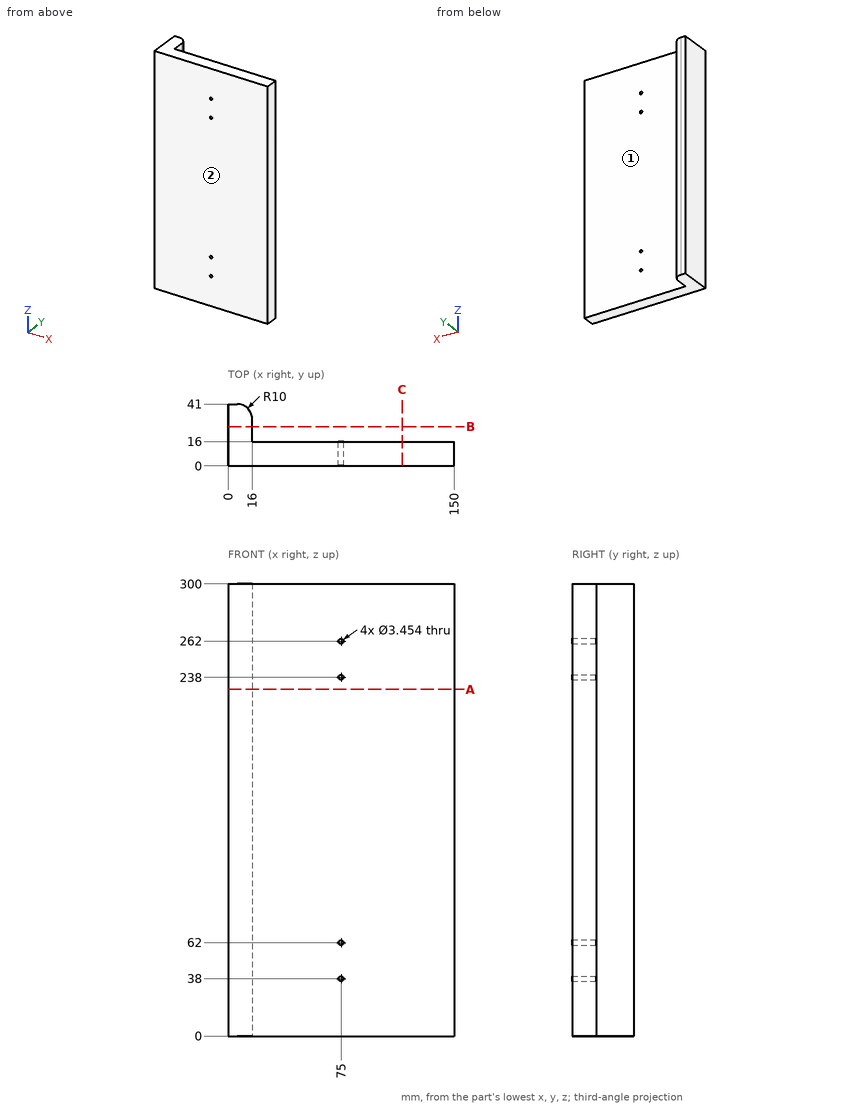
Study the drawing (mm; zero at the part's minimum x, y, z) and answer. A direction names the side the tool comes from. Round coordinates to 2 decimals unless told otherwise and drop trailing zeros. Write each loop counter-clockwise with the first axis right and the second up, starting at its lowest first coordinate (ties: lowest second). Pieces come first, ordered by that corner, then holes. Notation, with made-up numbers: (0.25, 89) -> (4.25, 89) arc R18 ccw to (4.25, 93) -> close; hole circle Ø6 at (13.25, 7.5). An arc over 180 degrees is marked (long way). Write item = value, one per line.
1) Section B-B on y = 26 is taken. Write down the section's boundary in (x, z).
Check values:
outline = (0, 0) -> (16, 0) -> (16, 300) -> (0, 300) -> close
2) Straight lines are drawn through the part: line 1 along Z through (x, y) = (75, 11); line 2 along X through (y, z) = (3, 238); line 3 along Y through (x, z) = (77, 148.5). For each, find the intervals that lie inside material, in ascending order. Write a range as [from, to].
Check values:
line_1 = [0, 36.27], [39.73, 60.27], [63.73, 236.27], [239.73, 260.27], [263.73, 300]
line_2 = [0, 73.27], [76.73, 150]
line_3 = [0, 16]
3) Given pin 1 (5.5 mm diameter, centred on x = 75, z = 62, fed in from +Y); pin 2 (3 mm diameter, centred on y = 29.5, z = 84.5, fed in from +X); pin 3 (2 mm diameter, centred on y = 34.5, z = 174.5, fed in from -X), each flat-ended and moving along its own axis, determine where each tip first touches the part or whether it passes through.
Check values:
pin_1 = 16
pin_2 = 16
pin_3 = 0
4) Which of the six approach directions +Z, -Z, +X, -X, +Y, -Y give full straight-line access (tool end or side, diameter ignored) to the marked faces 1 and 2?
Check values:
face_1 = +Z, -Z, +X, +Y
face_2 = +Z, -Z, +X, -X, -Y
5) Section A-A on z = 230 is taken. Write down the section's boundary in (x, y).
Check values:
outline = (0, 0) -> (150, 0) -> (150, 16) -> (16, 16) -> (16, 31) arc R10 ccw to (6, 41) -> (0, 41) -> close
